from build123d import *

# Parameters (mm, degrees)
SKETCH_1_W          = 70
SKETCH_1_H          = 20
EXTRUDE_1_DEPTH     = 4
SKETCH_2_R          = 2.1
CUT_EXTRUDE_1_DEPTH = 4
SKETCH_3_W          = 15
SKETCH_3_H          = 20
EXTRUDE_2_DEPTH     = 88
SKETCH_4_W          = 100
SKETCH_4_H          = 20
EXTRUDE_3_DEPTH     = 6
SKETCH_5_W          = 5
SKETCH_5_H          = 20
EXTRUDE_4_DEPTH     = 20
SKETCH_6_R          = 1.6
CUT_EXTRUDE_2_DEPTH = 95
CUT_EXTRUDE_START   = -20
SKETCH_6_2_R        = 1.6
CUT_EXTRUDE_3_DEPTH = 20
EXTRUDE_5_DEPTH     = 20
EXTRUDE_6_DEPTH     = 20
FILLET_1_R          = 3
FILLET_2_R          = 1


with BuildPart() as part:
    # 草图1 → 凸台-拉伸1 (new body)
    with BuildSketch(Plane.XY):
        with Locations((7.889344262, 6.686147681)):
            Rectangle(SKETCH_1_W, SKETCH_1_H)
    extrude(amount=EXTRUDE_1_DEPTH)

    # 草图2 → 切除-拉伸1 (cut)
    with BuildSketch(Plane.XY.offset(4)):
        with Locations((-14.610655738, 9.186147681)):
            Circle(SKETCH_2_R)
        with Locations((30.389344262, 9.186147681)):
            Circle(SKETCH_2_R)
    extrude(amount=-CUT_EXTRUDE_1_DEPTH, mode=Mode.SUBTRACT)

    # 草图3 → 凸台-拉伸2 (add)
    with BuildSketch(Plane.XY.offset(4)):
        with Locations((7.889344262, 6.686147681)):
            Rectangle(SKETCH_3_W, SKETCH_3_H)
    extrude(amount=EXTRUDE_2_DEPTH)

    # 草图4 → 凸台-拉伸3 (add)
    with BuildSketch(Plane.XY.offset(92)):
        with Locations((7.889344262, 6.686147681)):
            Rectangle(SKETCH_4_W, SKETCH_4_H)
    extrude(amount=EXTRUDE_3_DEPTH)

    # 草图5 → 凸台-拉伸4 (add)
    with BuildSketch(Plane.XY.offset(98)):
        with Locations((-39.610655738, 6.686147681)):
            Rectangle(SKETCH_5_W, SKETCH_5_H)
        with Locations((55.389344262, 6.686147681)):
            Rectangle(SKETCH_5_W, SKETCH_5_H)
    extrude(amount=EXTRUDE_4_DEPTH)

    # 草图6 → 切除-拉伸2 (cut)
    with BuildSketch(Plane(origin=(-37.110655738, 0, 0), x_dir=(0, 0, -1), z_dir=(1, 0, 0))):
        with Locations(Location((-101.5, 12.686147681, 0), (0, 0, 180))):
            Circle(SKETCH_6_R)
        with Locations(Location((-113.5, 0.686147681, 0), (0, 0, 180))):
            Circle(SKETCH_6_R)
    extrude(amount=CUT_EXTRUDE_2_DEPTH, mode=Mode.SUBTRACT)

    # 草图6<2> → 切除-拉伸3 (cut)
    with BuildSketch(Plane(origin=(-37.110655738, 0, 0), x_dir=(0, 0, -1), z_dir=(1, 0, 0)).offset(CUT_EXTRUDE_START)):
        with Locations(Location((-101.5, 12.686147681, 0), (0, 0, 180))):
            Circle(SKETCH_6_2_R)
        with Locations(Location((-113.5, 0.686147681, 0), (0, 0, 180))):
            Circle(SKETCH_6_2_R)
    extrude(amount=CUT_EXTRUDE_3_DEPTH, mode=Mode.SUBTRACT)

    # 草图7 → 凸台-拉伸5 (add)
    with BuildSketch(Plane.XZ.offset(3.313852319)):
        Polygon((0.389344262, 4), (0.389344262, 19.90041694), (-6.610655738, 4), align=None)
        Polygon((15.389344262, 4), (22.389344262, 4), (15.389344262, 19.90041694), align=None)
    extrude(amount=-EXTRUDE_5_DEPTH)

    # 草图8 → 凸台-拉伸6 (add)
    with BuildSketch(Plane.XZ.offset(3.313852319)):
        Polygon((-5.610655738, 92), (0.389344262, 82), (0.389344262, 92), align=None)
        Polygon((15.389344262, 82), (15.389344262, 92), (21.389344262, 92), align=None)
    extrude(amount=-EXTRUDE_6_DEPTH)

    # 圆角1
    fillet_1_edges = [part.edges().sort_by_distance(p)[0] for p in [
        (-6.610655738, 6.686147681, 4),
        (0.389344262, 6.686147681, 19.90041694),
        (15.389344262, 6.686147681, 19.90041694),
        (22.389344262, 6.686147681, 4),
        (-5.610655738, 6.686147681, 92),
        (0.389344262, 6.686147681, 82),
        (21.389344262, 6.686147681, 92),
        (15.389344262, 6.686147681, 82),
        (-42.110655738, 6.686147681, 92),
        (57.889344262, 6.686147681, 92),
    ]]
    fillet(fillet_1_edges, radius=FILLET_1_R)

    # 圆角2
    fillet_2_edges = [part.edges().sort_by_distance(p)[0] for p in [
        (-37.110655738, 6.686147681, 98),
        (52.889344262, 6.686147681, 98),
    ]]
    fillet(fillet_2_edges, radius=FILLET_2_R)


solid = part.part
For this review, take the finished solid that the model builds, in its own axes (mm). A direction names the side the tool comes from. Round coordinates to 2 decimals unless told otherwise and drop trailing zeros. Write each loop counter-clockwise with the first axis right and the second up, starting at its lowest first coordinate (ties: lowest second). Pieces come first, ordered by that corner, then holes. Notation, with made-up numbers: (-31.75, 31.5) - (-23.75, 31.5) arc R8 ccw to (-23.75, 41.5) - close; hole circle Ø10 at (-10, 61.25). An arc over 180 degrees is marked (long way). Use a Markdown table: item, result.
Q1. We need section A-A (z = 113.5). Give the boundary of the cut face in (x, y).
Derived:
| item | result |
|---|---|
| outline | (-42.11, -3.31) - (-37.11, -3.31) - (-37.11, -0.91) - (-42.11, -0.91) - close; (-42.11, 2.29) - (-37.11, 2.29) - (-37.11, 16.69) - (-42.11, 16.69) - close; (52.89, -3.31) - (57.89, -3.31) - (57.89, -0.91) - (52.89, -0.91) - close; (52.89, 2.29) - (57.89, 2.29) - (57.89, 16.69) - (52.89, 16.69) - close |
Q2. Clearance check with flat-ended pins moving along their axes: pin 1 (2 mm diameter, centred on y = 11, z = 43.5, fed in from -X); pin 2 (12 mm diameter, centred on y = 8, z = 25, fed in from +X); pin 3 (4 mm diameter, centred on x = -16.5, y = -1, fed in from +Z). State where each tip first meets the part, or that it passes through.
Derived:
| item | result |
|---|---|
| pin 1 | stops at x = 0.39 |
| pin 2 | stops at x = 15.79 |
| pin 3 | stops at z = 98 |
Q3. We need section B-B (x = 26). Give the boundary of the cut face in (y, z), plus the area to 3 significant figures.
Derived:
| item | result |
|---|---|
| outline | (-3.31, 0) - (16.69, 0) - (16.69, 4) - (-3.31, 4) - close; (-3.31, 92) - (16.69, 92) - (16.69, 98) - (-3.31, 98) - close |
| area | 200 mm2 |
Q4. Machinability: for faces 1 (the flat face through (42.889, 7, 2)), 2 (the flat face through (-27.111, 7, 2)), 3 (the cylindrical face through (-6.91, 6.83, 4.5)), 4 (the cylindrical face through (22.728, 6.826, 4.474)), which of the approach directions +Z, -Z, +X, -X, +Y, -Y give a long, thin tool a straight path to every point of the face, cutting with its end or side? Answer none if there is none.
Derived:
| item | result |
|---|---|
| face 1 | -Z, +X, +Y, -Y |
| face 2 | -Z, -X, +Y, -Y |
| face 3 | -X, +Y, -Y |
| face 4 | +X, +Y, -Y |
Q5. The part is to be moulded in two halves that separate along Y. For faces 5 (the cylindrical face through (55.35, 12.62, 99.9)), 6 (the flat face through (18.199, 6.546, 86.683)), say which applies: pulls with the +Y half, pulls with the -Y half, needs draft (parallel to the pull), parting line crosses it, or undercut.
Derived:
| item | result |
|---|---|
| face 5 | undercut |
| face 6 | needs draft |
Q6. We need section C-C (z = 30.5). Give the boundary of the cut face in (x, y), plus the area to 3 significant figures.
Derived:
| item | result |
|---|---|
| outline | (0.39, -3.31) - (15.39, -3.31) - (15.39, 16.69) - (0.39, 16.69) - close |
| area | 300 mm2 |
Q7. Wall thickness on line 1 along Y through (x, z) = (54.5, 101.5); line 2 along Z through (x, y) = (37, 16.25); line 3 along Y through (x, z) = (56.3, 113.5): over which ranges is each line inside the solid? List them lowest first.
Derived:
| item | result |
|---|---|
| line 1 | y = -3.31 to 11.09, 14.29 to 16.69 |
| line 2 | z = 0 to 4, 92 to 98 |
| line 3 | y = -3.31 to -0.91, 2.29 to 16.69 |
Q8. We need section D-D (x = 45.5). Give the boundary of the cut face in (y, z), plus the area to 3 significant figures.
Derived:
| item | result |
|---|---|
| outline | (-3.31, 92) - (16.69, 92) - (16.69, 98) - (-3.31, 98) - close |
| area | 120 mm2 |
